Input: part model. Units: mm. Frame: model coordinates. A direction names the side the tool comes from. Coordinates: 2 decimals unless noted, no trailing zeros. Loops run counter-clockwise (first coordinate to the right, second up) from the corner with the lowest first, then second, coordinate; pieces in that order, holes last. Notation, with made-up numbers: (-11, -13) -> (37, -13) arc R22 ccw to (37, 2) -> close; hole circle Ø4 at (-24.75, 48). An arc over 180 degrees is marked (long way). Answer as a JSON object with one key per item and string values.
from build123d import *

# Parameters (mm, degrees)
SKETCH_1_W               = 15
SKETCH_1_H               = 15
SKETCH_1_W_2             = 12
SKETCH_1_H_2             = 12
EXTRUDE_1_DEPTH          = 160
SKETCH_3_R               = 6
CUT_EXTRUDE_3_DEPTH      = 161.876505432
SKETCH_7_R               = 2
CUT_EXTRUDE_4_DEPTH      = 161.876505432
CUT_EXTRUDE_5_DEPTH      = 161.876505432
CUT_EXTRUDE_5_DEPTH_BACK = 161.876505432
SKETCH_12_R              = 1.6
SKETCH_13_W              = 15
SKETCH_13_H              = 15
SKETCH_13_W_2            = 12
SKETCH_13_H_2            = 12
EXTRUDE_1_2_DEPTH        = 10


with BuildPart() as part:
    # ｽｹｯﾁ1 → Extrude 1 (new body)
    with BuildSketch(Plane.XY):
        Rectangle(SKETCH_1_W, SKETCH_1_H)
        Rectangle(SKETCH_1_W_2, SKETCH_1_H_2, mode=Mode.SUBTRACT)
    extrude(amount=EXTRUDE_1_DEPTH)

    # ｽｹｯﾁ3 → ｶｯﾄ - 押し出し3 (cut, through all)
    with BuildSketch(Plane.XZ.offset(7.5)):
        with Locations(Location((0, 140, 0), (0, 0, 180))):
            Circle(SKETCH_3_R)
    extrude(amount=-CUT_EXTRUDE_3_DEPTH, mode=Mode.SUBTRACT)

    # ｽｹｯﾁ7 → ｶｯﾄ - 押し出し4 (cut, through all)
    with BuildSketch(Plane.ZY.offset(7.5)):
        with Locations((140, 0)):
            Circle(SKETCH_7_R)
    extrude(amount=-CUT_EXTRUDE_4_DEPTH, mode=Mode.SUBTRACT)

    # ｽｹｯﾁ12 → ｶｯﾄ - 押し出し5 (cut, two sides: drawn at the far end of the back side and taken through both)
    with BuildSketch(Plane(origin=(7.5, 0, 0), x_dir=(0, 0, -1), z_dir=(1, 0, 0)).offset(-CUT_EXTRUDE_5_DEPTH_BACK)):
        with Locations((-38, 0)):
            Circle(SKETCH_12_R)
        with Locations((-62, 0)):
            Circle(SKETCH_12_R)
    extrude(amount=CUT_EXTRUDE_5_DEPTH + CUT_EXTRUDE_5_DEPTH_BACK, mode=Mode.SUBTRACT)

    # ｽｹｯﾁ13 → Extrude 1 2 (add)
    with BuildSketch(Plane.XY.offset(160)):
        Rectangle(SKETCH_13_W, SKETCH_13_H)
        Rectangle(SKETCH_13_W_2, SKETCH_13_H_2, mode=Mode.SUBTRACT)
    extrude(amount=EXTRUDE_1_2_DEPTH)


solid = part.part
1. Section query C-C (y = 0). Count the separate pieces of the cut face and the enclosed holes in it, plus the area to 3 significant figures.
Reply:
{"separate pieces": "8", "enclosed holes": "0", "area": "479 mm2"}
2. Pin query (flat end, axial travel): P1, Ø7, axis at x = 0, z = 140, coming from the -Y side. Return the tip coordinate at first contact, or that it passes through.
Reply:
{"P1": "passes through"}
3. Mould query, pull axis Y, two halves, no side actions, for faces 1 (the face through (0, 7.5, 84)), 2 (the face through (-7, 0, 0)), 3 (the face through (0, 6, 69)). Classes: pulls with the +Y half, pulls with the -Y half, needs draft (parallel to the pull), parting line crosses it, or undercut.
Reply:
{"face 1": "pulls with the +Y half", "face 2": "needs draft", "face 3": "undercut"}
4. Section query A-A (z = 38). Return loops of the section in (x, y), plus the area to 3 significant figures.
Reply:
{"outline": "(-7.5, -7.5) -> (7.5, -7.5) -> (7.5, -1.6) -> (6, -1.6) -> (6, -6) -> (-6, -6) -> (-6, -1.6) -> (-7.5, -1.6) -> close; (-7.5, 1.6) -> (-6, 1.6) -> (-6, 6) -> (6, 6) -> (6, 1.6) -> (7.5, 1.6) -> (7.5, 7.5) -> (-7.5, 7.5) -> close", "area": "71.4 mm2"}
5. Section query D-D (z = 136). Return loops of the section in (x, y).
Reply:
{"outline": "(-7.5, -7.5) -> (-4.47, -7.5) -> (-4.47, -6) -> (-6, -6) -> (-6, 6) -> (-4.47, 6) -> (-4.47, 7.5) -> (-7.5, 7.5) -> close; (4.47, -7.5) -> (7.5, -7.5) -> (7.5, 7.5) -> (4.47, 7.5) -> (4.47, 6) -> (6, 6) -> (6, -6) -> (4.47, -6) -> close"}
6. Line query: line 1 along Y through (x, z) = (6.4, 38); line 2 along X through (y, z) = (4.25, 22). Output: solid intervals per line, ascending.
Reply:
{"line 1": "y = -7.5 to -1.6, 1.6 to 7.5", "line 2": "x = -7.5 to -6, 6 to 7.5"}
7. Access query for faces 4 (the face through (-6.76, 1.08, 39.18)), 5 (the face through (0, 6, 158)). Directions: +Z, -Z, +X, -X, +Y, -Y. A direction counts if a zero-diameter tool reaches every point of the face in a straight line with its end or side. Return the directions, or none.
Reply:
{"face 4": "+X, -X", "face 5": "+Z, -Z"}
8. Section query B-B (x = 0). Return loops of the section in (y, z).
Reply:
{"outline": "(-7.5, 0) -> (-6, 0) -> (-6, 134) -> (-7.5, 134) -> close; (-7.5, 146) -> (-6, 146) -> (-6, 170) -> (-7.5, 170) -> close; (6, 0) -> (7.5, 0) -> (7.5, 134) -> (6, 134) -> close; (6, 146) -> (7.5, 146) -> (7.5, 170) -> (6, 170) -> close"}
